Work out the finished part from the listing and answer in its coordinate system (mm). Face numbers are marked on the shaded views. A direction names the side the tool comes from. Round coordinates to 2 decimals unless told otherwise and drop trailing zeros. Order: outer loops, then holes, each group sorted by start corner. A loop starts at its lowest first (then second) coordinate and runs counter-clockwise, first axis right, second up. Notation, with made-up numbers: (-26, 57) - (12, 57) arc R23 ccw to (12, 77) - close; hole circle Ø5 at (10, -0.5). An arc over 180 degrees is marked (long way). Use one line per item in the form item = value. Start each with the question number.
Q1. The part is cut by section A-A on z = 22. Determine the outline of the cut face in (x, y).
Q2. The part is cut by section B-B on y = 2.5. Determine the outline of the cut face in (x, z), plus the area to 3 significant figures.
Q3. Find the intervals of material crossed by line 1 (Y direction, x = -20, z = 43); line 2 (Z direction, x = 58, y = -31), in increasing order. Write a range as [from, to].
Q4. The part is cut by section C-C on x = -15. Determine the outline of the cut face in (y, z).
Q5. For a pull along Z with two mould halves and no side action, classify the marked faces 1, 2 and 3 as +Z half, -Z half, draft (parallel to the pull), parting line (faces both ways), or undercut.
Q6. Which of the six approach directions +Z, -Z, +X, -X, +Y, -Y give full straight-line access (tool end or side, diameter ignored) to the marked faces 4 and 5?
Q7. Given P1, Ø3, axis at x = 94.43, y = -58.38, coming from the -Z side; P2, Ø6.5, axis at x = 43.63, y = -32.98, coming from the +Z side, each flat-ended and moving along its own axis, determine where each tip first touches the part or whether it passes through.
from build123d import *

# Parameters (mm, degrees)
F0_W     = 304.8
F0_H     = 101.6
F1_DEPTH = 50.8
F2_W     = 96.52
F2_H     = 45.72
F3_DEPTH = 304.801
F5_D     = 5.1054


with BuildPart() as f1:
    # F0 (on Top) → F1 (new body)
    with BuildSketch(Plane.XY):
        with Locations((5.528525, -20.282418)):
            Rectangle(F0_W, F0_H)
    extrude(amount=F1_DEPTH)

    # F2 (on face) → F3 (cut, through all)
    with BuildSketch(Plane(origin=(-146.871475, 0, 0), x_dir=(0, -1, 0), z_dir=(-1, 0, 0))):
        with Locations((20.282418, 25.4)):
            Rectangle(F2_W, F2_H)
    extrude(amount=-F3_DEPTH, mode=Mode.SUBTRACT)

    # F5 (through all)
    with Locations(Plane.XY.offset(50.8)):
        with Locations((145.228525, -58.382418), (43.628525, -58.382418), (-57.971475, -58.382418), (94.428525, -32.982418), (-7.171475, -32.982418), (119.828525, -7.582418), (69.028525, 17.817582), (18.228525, -7.582418), (-32.571475, 17.817582), (69.028525, -58.382418), (-32.571475, -58.382418), (145.228525, 17.817582), (43.628525, 17.817582), (-57.971475, 17.817582), (94.428525, -58.382418), (-7.171475, -58.382418), (119.828525, -32.982418), (69.028525, -7.582418), (18.228525, -32.982418), (-32.571475, -7.582418), (145.228525, -7.582418), (43.628525, -7.582418), (-57.971475, -7.582418), (119.828525, 17.817582), (-83.371475, -7.582418), (18.228525, 17.817582), (-83.371475, -32.982418), (-83.371475, -58.382418), (94.428525, 17.817582), (-7.171475, 17.817582), (-134.171475, 17.817582), (119.828525, -58.382418), (18.228525, -58.382418), (69.028525, -32.982418), (-32.571475, -32.982418), (-134.171475, -7.582418), (-134.171475, -32.982418), (145.228525, -32.982418), (43.628525, -32.982418), (-134.171475, -58.382418), (-57.971475, -32.982418), (-108.771475, 17.817582), (-108.771475, -7.582418), (-108.771475, -32.982418), (-108.771475, -58.382418), (-83.371475, 17.817582), (94.428525, -7.582418), (-7.171475, -7.582418)):
            Hole(F5_D / 2)


solid = f1.part
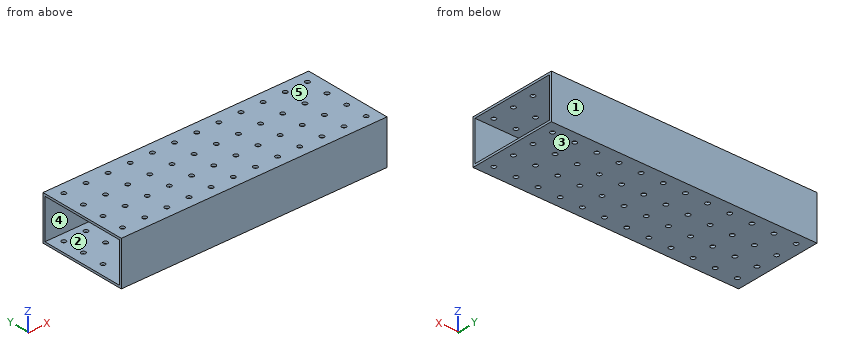
Found:
q1.outline = (-146.87, -71.08) - (157.93, -71.08) - (157.93, -68.54) - (-146.87, -68.54) - close; (-146.87, 27.98) - (157.93, 27.98) - (157.93, 30.52) - (-146.87, 30.52) - close
q2.outline = (-146.87, 0) - (157.93, 0) - (157.93, 2.54) - (-146.87, 2.54) - close; (-146.87, 48.26) - (157.93, 48.26) - (157.93, 50.8) - (-146.87, 50.8) - close
q2.area = 1,550 mm²
q3.line_1 = [-71.08, -68.54], [27.98, 30.52]
q3.line_2 = [0, 2.54], [48.26, 50.8]
q4.outline = (-71.08, 0) - (30.52, 0) - (30.52, 50.8) - (-71.08, 50.8) - close; hole (-68.54, 2.54) - (27.98, 2.54) - (27.98, 48.26) - (-68.54, 48.26) - close
q5.face_1 = draft
q5.face_2 = undercut
q5.face_3 = -Z half
q6.face_4 = +X, -X
q6.face_5 = +Z, +X, -X, +Y, -Y
q7.P1 = through
q7.P2 = 50.8
